Work out the finished part from the listing and answer in its coordinate system (mm). Give positions to 0.01 mm unless a question says otherwise; leave off trailing zeros. Loops run counter-clockwise (first coordinate to the right, second up) from the corner with the lowest first, then second, coordinate; pieces in that order, holes last. Notation, with made-up numbers: (35.5, -27) - (43.5, -27) arc R25 ccw to (43.5, -3) - close; hole circle Ø8 at (86.5, -21). An arc over 180 degrees is marked (long way). One line per item, written item: value.
Autodesk Inventor part; units mm, degrees
ref_plane "YZ Plane" through (0, 0, 0) normal (1, 0, 0) x (0, 1, 0)
ref_plane "XZ Plane" through (0, 0, 0) normal (0, 1, 0) x (-1, 0, 0)
ref_plane "XY Plane" through (0, 0, 0) normal (0, 0, 1) x (1, 0, 0)
sketch "Sketch1" plane through (0, 0, 0) normal (0, 0, 1) x (1, 0, 0)
  line L0 (-85, 60) -> (85, 60)
  line L1 (85, 60) -> (85, -60)
  line L2 (85, -60) -> (-85, -60)
  line L3 (-85, -60) -> (-85, 60)
  line L4 (-85, 60) -> (85, -60) construction
  line L5 (85, 60) -> (-85, -60) construction
  circle A0 centre (-25, 0) radius 30
  line L6 (0, 60) -> (0, -60) construction
  arc A1 (-25, 60) -> (-25, -60) centre (-25, 0) ccw
  line L7 (85, 17.2792) -> (7.7208, -60)
  line L8 (85, 17.2792) -> (42.2792, 60)
  point P0 (0, 0)
  point P1 (-85, 0)
  dimension "d0" = 170
  dimension "d1" = 120
  dimension "d13" = 60
  dimension "d14" = 60
  dimension "d17" = 45
  dimension "d18" = 90
extrude "Plate1" add sketch "Sketch1" along normal blind 4 contours L0 L8 L7 L2 A1
fillet "Corner Round1" radius 2 3 edges at (85, 17.2792, 2) (42.2792, 60, 2) (7.7208, -60, 2)
equation "\"d2\" = Thickness"
equation "\"BendRadius\" = Thickness"
equation "\"BendReliefWidth\" = Thickness"
equation "\"BendReliefDepth\" = 0.5 * Thickness"
equation "\"CornerReliefSize\" = 4 * Thickness"
equation "\"MinimumRemnant\" = 2 * Thickness"
equation "\"TransitionRadius\" = BendRadius"
equation "\"JacobiRadiusSize\" = BendRadius"
equation "\"GapSize\" = Thickness"
properties part number "ухо"
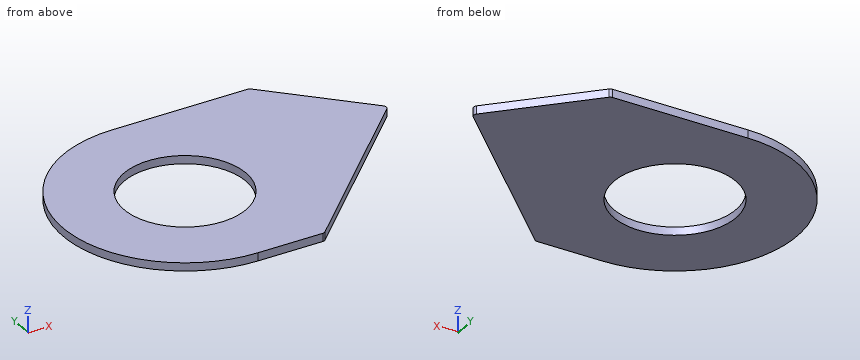
1. Section D-D (x = 49) is taken. Write down the section's boundary in (y, z).
Output:
outline: (-18.72, 0) - (53.28, 0) - (53.28, 4) - (-18.72, 4) - close
2. Flat-ended cylindrical pins translate along their axes: pin 1 Ø1.5 at (y, z) = (35.5, 0.5) entering from -X; pin 2 Ø1.5 at (y, z) = (-36, 2.5) entering from +X; pin 3 Ø1.5 at (y, z) = (35, 3) entering from -X. Find the tip coordinate at first contact, or state that the pin passes through.
Output:
pin 1: stops at x = -73.91
pin 2: stops at x = 32.47
pin 3: stops at x = -74.26
3. Section A-A (y = -18) is taken. Write down the section's boundary in (x, z).
Output:
outline: (-82.24, 0) - (-49, 0) - (-49, 4) - (-82.24, 4) - close; (-1, 0) - (49.72, 0) - (49.72, 4) - (-1, 4) - close
4. Find the intervals of material crossed by line 1 along Y through (x, z) = (-25, 1.3); line 2 along Y through (x, z) = (-41, 1.25); line 3 along X through (y, z) = (6, 2.35), in increasing order.
Output:
line 1: y = -60 to -30, 30 to 60
line 2: y = -57.83 to -25.38, 25.38 to 57.83
line 3: x = -84.7 to -54.39, 4.39 to 73.72
5. Section B-B (z = 3.35) is taken. Write down the section's boundary in (x, y), and give its area (3 significant figures).
Output:
outline: (-25, -60) - (6.89, -60) arc R2 ccw to (8.31, -59.41) - (83.59, 15.86) arc R2 ccw to (83.59, 18.69) - (42.86, 59.41) arc R2 ccw to (41.45, 60) - (-25, 60) arc R60 ccw to start; hole circle Ø60 at (-25, 0)
area: 12,100 mm²
6. Section C-C (x = -45) is taken. Write down the section's boundary in (y, z), and give its area (3 significant figures).
Output:
outline: (-56.57, 0) - (-22.36, 0) - (-22.36, 4) - (-56.57, 4) - close; (22.36, 0) - (56.57, 0) - (56.57, 4) - (22.36, 4) - close
area: 274 mm²
